```python
from build123d import *

# Parameters (mm, degrees)
F1_DEPTH = 25.4
F2_R     = 1.7272
F3_DEPTH = 4.7625
F4_R     = 3.96875


with BuildPart() as f1:
    # F0 (on Top) → F1 (new body)
    with BuildSketch(Plane.XY):
        with BuildLine():
            ThreePointArc((-10.4, 0), (-5.2, 13.934491), (0, 0))
            Line((0, 0), (0, -14.480139))
            Line((0, -14.480139), (2.7375, -14.480139))
            Line((2.7375, -14.480139), (2.7375, -1.780139))
            ThreePointArc((2.7375, -1.780139), (-5.2, 17.109491), (-13.1375, -1.780139))
            Line((-13.1375, -1.780139), (-13.1375, -14.480139))
            Line((-13.1375, -14.480139), (-10.4, -14.480139))
            Line((-10.4, -14.480139), (-10.4, 0))
        make_face()
    extrude(amount=F1_DEPTH)

    # F2 (on face) → F3 (join)
    with BuildSketch(Plane.XY.offset(25.4)):
        with BuildLine():
            Line((-19.832804, -8.635813), (-13.1375, -8.635813))
            Line((-13.1375, -8.635813), (-13.1375, -1.780139))
            ThreePointArc((-13.1375, -1.780139), (-5.2, 17.109491), (2.7375, -1.780139))
            Line((2.7375, -1.780139), (2.7375, -8.635813))
            Line((2.7375, -8.635813), (9.432804, -8.635813))
            Line((9.432804, -8.635813), (9.432804, 20.629796))
            Line((9.432804, 20.629796), (-19.832804, 20.629796))
            Line((-19.832804, 20.629796), (-19.832804, -8.635813))
        make_face()
        with Locations((-15.864054, -4.667063)):
            Circle(F2_R, mode=Mode.SUBTRACT)
        with Locations((5.464054, -4.667063)):
            Circle(F2_R, mode=Mode.SUBTRACT)
        with Locations((-15.864054, 16.661046)):
            Circle(F2_R, mode=Mode.SUBTRACT)
        with Locations((5.464054, 16.661046)):
            Circle(F2_R, mode=Mode.SUBTRACT)
        with BuildLine():
            Line((-13.1375, -8.635813), (-13.1375, -14.480139))
            Line((-13.1375, -14.480139), (-10.4, -14.480139))
            Line((-10.4, -14.480139), (-10.4, 0))
            ThreePointArc((-10.4, 0), (-8.496127, 13.217757), (2.7375, 5.996991))
            ThreePointArc((2.7375, 5.996991), (2.020765, 2.700864), (0, 0))
            Line((0, 0), (0, -14.480139))
            Line((0, -14.480139), (2.7375, -14.480139))
            Line((2.7375, -14.480139), (2.7375, -8.635813))
            Line((2.7375, -8.635813), (2.7375, -1.780139))
            ThreePointArc((2.7375, -1.780139), (-5.2, 17.109491), (-13.1375, -1.780139))
            Line((-13.1375, -1.780139), (-13.1375, -8.635813))
        make_face()
        with BuildLine():
            Line((-10.4, 0), (-10.4, -14.480139))
            Line((-10.4, -14.480139), (0, -14.480139))
            Line((0, -14.480139), (0, 0))
            ThreePointArc((0, 0), (-5.2, -1.940509), (-10.4, 0))
        make_face()
    extrude(amount=F3_DEPTH)

    # F4
    f4_edges = [f1.edges().sort_by_distance(p)[0] for p in [
        (-19.832804, -8.635813, 27.78125),
        (9.432804, -8.635813, 27.78125),
        (9.432804, 20.629796, 27.78125),
        (-19.832804, 20.629796, 27.78125),
    ]]
    fillet(f4_edges, radius=F4_R)


solid = f1.part
```
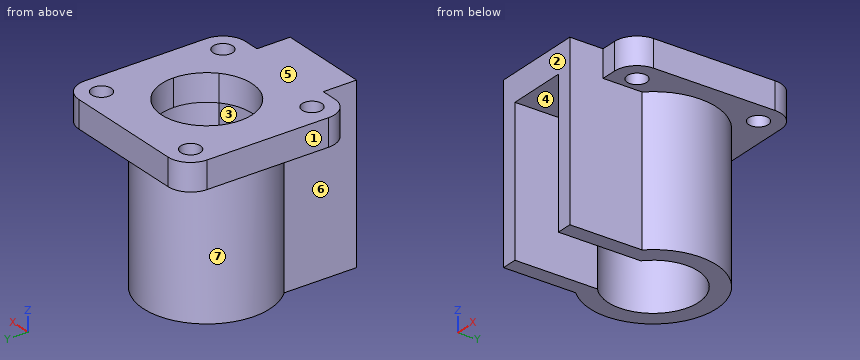
The model under review builds one solid part; all positions refer to its coordinate system, in mm. Face numbers are marked on the shaded views. A direction names the side the tool comes from. Round coordinates to 2 decimals unless told otherwise and drop trailing zeros. Order: outer loops, then holes, each group sorted by start corner. A loop starts at its lowest first (then second) coordinate and runs counter-clockwise, first axis right, second up.
(1) For P1, Ø3, axis at x = -15.86, y = -4.67, coming from the -Z side; P2, Ø12, axis at y = -5.5, z = 14, coming from the +X side; P3, Ø6.5, axis at y = -6.5, z = 11, coming from the +X side; P4, Ø3, axis at x = 6.5, z = 9.5, coming from the -Y side, all flat-tipped, find the tip position at first contact; note any pin that passes through.
Working result:
P1: passes through
P2: stops at x = 4.46
P3: stops at x = 2.74
P4: stops at y = 1.59
(2) Mouldability with a two-part tool opening along X and no side actions: class the marked faces 1, 2 and 3 as released by +X, released by -X, zero draft, split by the parting line, or undercut.
Working result:
face 1: released by -X
face 2: zero draft
face 3: undercut
(3) Take a section at C-C, the plane y = -3.5. State the section outline as (x, z) points.
Working result:
outline: (-19.83, 25.4) - (-17.14, 25.4) - (-17.14, 30.16) - (-19.83, 30.16) - close; (-14.59, 25.4) - (-13.14, 25.4) - (-13.14, 0) - (-10.4, 0) - (-10.4, 25.4) - (0, 25.4) - (0, 0) - (2.74, 0) - (2.74, 25.4) - (4.19, 25.4) - (4.19, 30.16) - (-14.59, 30.16) - close; (6.74, 25.4) - (9.43, 25.4) - (9.43, 30.16) - (6.74, 30.16) - close
(4) Take a section at B-B, the plane z = 27.5. State the section outline as (x, y) points (1 decimal).
Working result:
outline: (-19.8, -4.7) arc R4 ccw to (-15.9, -8.6) - (-13.1, -8.6) - (-13.1, -14.5) - (2.7, -14.5) - (2.7, -8.6) - (5.5, -8.6) arc R4 ccw to (9.4, -4.7) - (9.4, 16.7) arc R4 ccw to (5.5, 20.6) - (-15.9, 20.6) arc R4 ccw to (-19.8, 16.7) - close; hole circle Ø3.5 at (-15.9, -4.7); hole circle Ø3.5 at (-15.9, 16.7); hole (-10.4, 0) arc R7.9 ccw to (0, 0) arc R7.9 ccw to (2.7, 6) arc R7.9 ccw (long way) to start; hole circle Ø3.5 at (5.5, -4.7); hole circle Ø3.5 at (5.5, 16.7)
(5) Take a section at D-D, the plane z = 21. State the section outline as (x, y) points (1 decimal).
Working result:
outline: (-13.1, -14.5) - (-10.4, -14.5) - (-10.4, 0) arc R7.9 cw (long way) to (0, 0) - (0, -14.5) - (2.7, -14.5) - (2.7, -1.8) arc R11.1 ccw (long way) to (-13.1, -1.8) - close
(6) Wall thickness on L1, parallel to X at y = -4, z = 22; L2, parallel to Z at x = -15.5, y = -6.5; L3, parallel to X at y = 10, z = 18.5: over which ranges is each line inside the solid? List them lowest first.
Working result:
L1: x = -13.14 to -10.4, 0 to 2.74
L2: z = 25.4 to 30.16
L3: x = -15.57 to -12.05, 1.65 to 5.17
(7) Take a section at A-A, the plane x = -5.2. State the section outline as (y, z) points, plus the area to 3 significant figures.
Working result:
outline: (-14.48, 25.4) - (-1.94, 25.4) - (-1.94, 30.16) - (-14.48, 30.16) - close; (13.93, 0) - (17.11, 0) - (17.11, 25.4) - (20.63, 25.4) - (20.63, 30.16) - (13.93, 30.16) - close
area: 172 mm2
(8) Tool access review of the marked faces 4, 5, 6 and 7: name each direction out of +Z, -Z, +X, -X, +Y, -Y from which nothing blocks a thin tool from reaching the whole face with its end or side.
Working result:
face 4: -Z, -Y
face 5: +Z, +X, -X, +Y, -Y
face 6: -Z, -X, -Y
face 7: -Z
